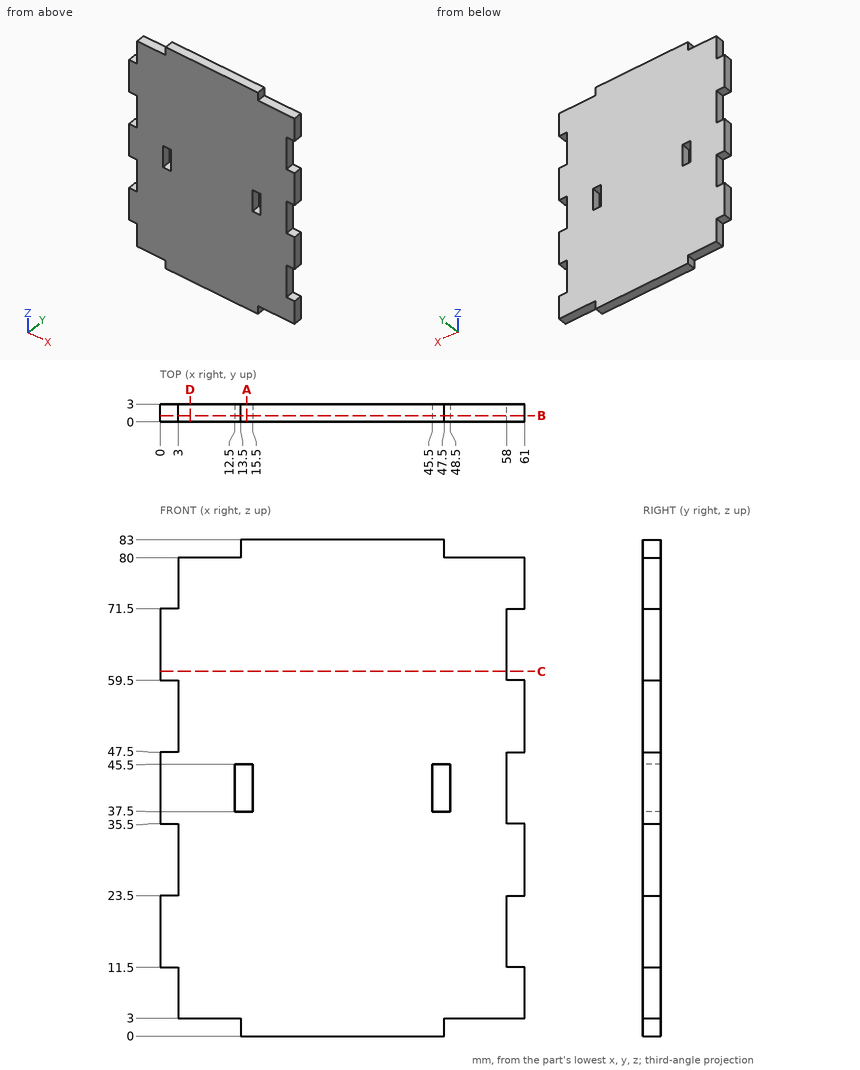
For this review, use the dimensioned drawing (mm, ordinates from the lowest corner) and the shaded views. Give positions to 0.01 mm unless a question says otherwise; leave off trailing zeros. Write each loop counter-clockwise with the first axis right and the second up, starting at its lowest first coordinate (ties: lowest second). Pieces come first, ordered by that corner, then holes.
(1) Consider section B-B, the plane y = 1.05. Give the number of separate pieces and of enclosed holes in the cut face, and give its area (3 significant figures).
(2) For P1, Ø1.5, axis at x = 59.5, y = 1, coming from the -Z side; P2, Ø1.5, axis at y = 2, z = 81.5, coming from the -X side; P3, Ø0.9, axis at y = 1, z = 64, coming from the +X side, all flat-tipped, find the tip position at first contact; note any pin that passes through.
(3) To check wall thickness, follow L1, parallel to Z at x = 58.5, y = 1.8; L2, parallel to Z at x = 14, y = 2.2; L3, parallel to X at y = 0.25, z = 67. State the ranges of each line that lie inside material, in increasing order.
(4) Consider section A-A, the plane x = 14.5. Give the boundary of the cut face in (y, z), and give its area (3 significant figures).
(5) Consider section D-D, the plane x = 5. Give the boundary of the cut face in (y, z).
(6) Consider section C-C, the plane z = 61. Give the boundary of the cut face in (x, y).
Returned:
1. separate pieces: 1
1. enclosed holes: 2
1. area: 4,620 mm2
2. P1: stops at z = 3
2. P2: stops at x = 13.5
2. P3: stops at x = 58
3. L1: z = 3 to 11.5, 23.5 to 35.5, 47.5 to 59.5, 71.5 to 80
3. L2: z = 0 to 37.5, 45.5 to 83
3. L3: x = 0 to 58
4. outline: (0, 0) - (3, 0) - (3, 37.5) - (0, 37.5) - close; (0, 45.5) - (3, 45.5) - (3, 83) - (0, 83) - close
4. area: 225 mm2
5. outline: (0, 3) - (3, 3) - (3, 80) - (0, 80) - close
6. outline: (0, 0) - (58, 0) - (58, 3) - (0, 3) - close
